Part model, mm, in its own coordinate system. Face numbers are marked on the shaded views. A direction names the side the tool comes from. Coordinates: 2 decimals unless noted, no trailing zeros. Loops run counter-clockwise (first coordinate to the right, second up) from the corner with the lowest first, then second, coordinate; pieces in that order, holes last. Notation, with made-up numbers: M 76.5,50.25 L 94.5,50.25 A10 ccw 94.5,68.25 Z; hole C 67.25,-1 d4. An arc over 180 degrees is marked long. Answer as CSV lines item,"result". Start each with the question number.
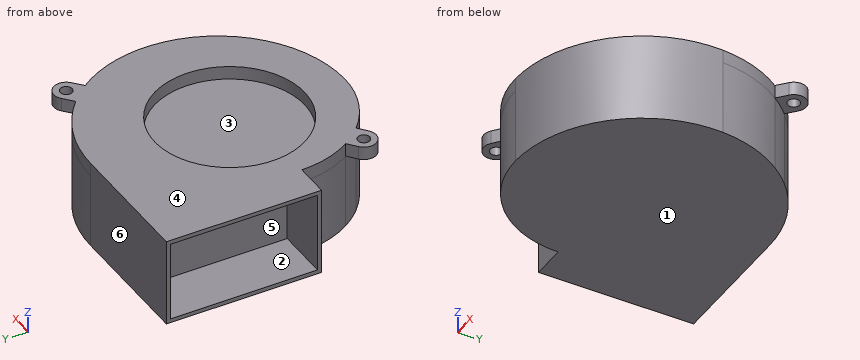
from build123d import *
from build123d.topology import SkipClean

# Parameters (mm, degrees)
SKETCH2_R           = 2.25
SKETCH2_R_2         = 28
BOSS_EXTRUDE1_DEPTH = 5
SKETCH5_R           = 28
BOSS_EXTRUDE3_DEPTH = 28
SKETCH6_W           = 30
SKETCH6_H           = 55
CUT_EXTRUDE1_DEPTH  = 20


with BuildPart() as part:
    # Sketch2 → Boss-Extrude1 (new body)
    # profile 1 of 3: a face of its own
    with BuildSketch(Plane.XY):
        with BuildLine():
            Line((35.933927487, 42.495954711), (32.250401879, 39.26537607))
            ThreePointArc((32.250401879, 39.26537607), (35.489083713, 35.92080567), (38.382546905, 32.273466648))
            Line((38.382546905, 32.273466648), (42.066072513, 35.504045289))
            ThreePointArc((42.066072513, 35.504045289), (42.495954711, 42.066072513), (35.933927487, 42.495954711))
        make_face()
        with Locations((39, 39)):
            Circle(SKETCH2_R, mode=Mode.SUBTRACT)
    # profile 2 of 3: a face of its own
    with BuildSketch(Plane.XY):
        with BuildLine():
            ThreePointArc((-25.556282339, -32.755867263), (-28.716218004, -29.331927128), (-31.420793753, -25.538007062))
            Line((-31.420793753, -25.538007062), (-34.932255707, -28.391069899))
            ThreePointArc((-34.932255707, -28.391069899), (-35.608930101, -34.932255707), (-29.067744293, -35.608930101))
            Line((-29.067744293, -35.608930101), (-25.556282339, -32.755867263))
        make_face()
        with Locations((-32, -32)):
            Circle(SKETCH2_R, mode=Mode.SUBTRACT)
    # profile 3 of 3: a face of its own
    with BuildSketch(Plane.XY):
        with BuildLine():
            ThreePointArc((0, -43), (-26.162950904, -32.162950904), (-37, -6))
            Line((-37, -6), (-50, -6))
            Line((-50, -6), (-50, 52))
            Line((-50, 52), (0, 52))
            ThreePointArc((0, 52), (32.250401879, 39.26537607), (47.1, 7.932509882))
            ThreePointArc((47.1, 7.932509882), (34.50998509, -27.669026021), (0, -43))
        make_face()
        Circle(SKETCH2_R_2, mode=Mode.SUBTRACT)
    extrude(amount=-BOSS_EXTRUDE1_DEPTH)

    # Sketch5 → Boss-Extrude3 (add)
    # profile 1 of 2: a face of its own
    with SkipClean():  # the faces are left unmerged after this step: merging them gives an invalid solid
        with BuildSketch(Plane.XY.offset(-5)):
            with BuildLine():
                ThreePointArc((32.250401879, 39.26537607), (17.336803829, 48.701069191), (0, 52))
                Line((0, 52), (-50, 52))
                Line((-50, 52), (-50, -6))
                Line((-50, -6), (-37, -6))
                ThreePointArc((-37, -6), (-35.577867902, -16.159493864), (-31.420793753, -25.538007062))
                ThreePointArc((-31.420793753, -25.538007062), (-28.716218004, -29.331927128), (-25.556282339, -32.755867263))
                ThreePointArc((-25.556282339, -32.755867263), (-13.766497581, -40.34360995), (0, -43))
                ThreePointArc((0, -43), (34.50998509, -27.669026021), (47.1, 7.932509882))
                ThreePointArc((47.1, 7.932509882), (44.44026328, 20.711463284), (38.382546905, 32.273466648))
                ThreePointArc((38.382546905, 32.273466648), (35.489083713, 35.92080567), (32.250401879, 39.26537607))
            make_face()
            Circle(SKETCH5_R, mode=Mode.SUBTRACT)
        # profile 2 of 2: a face of its own
        with BuildSketch(Plane.XY.offset(-5)):
            Circle(SKETCH5_R)
        extrude(amount=-BOSS_EXTRUDE3_DEPTH)

    # Sketch6 → Cut-Extrude1 (cut)
    with SkipClean():  # the faces are left unmerged after this step: merging them gives an invalid solid
        with BuildSketch(Plane.ZY.offset(50)):
            with Locations((-16.5, 23)):
                Rectangle(SKETCH6_W, SKETCH6_H)
        extrude(amount=-CUT_EXTRUDE1_DEPTH, mode=Mode.SUBTRACT)


solid = part.part
Q1. Flat gauge pins, fed straight in: P1, Ø9, axis at x = 37, y = 36, coming from the -Z side; P2, Ø5.5, axis at x = -30.5, y = -33.5, coming from the -Z side; P3, Ø4, axis at y = -2.5, z = -18.5, coming from the +X side; P4, Ø6, axis at x = 11.5, z = -15, coming from the +Y side. Where does each tip first touch, or does it go through?
Q2. Slice it at B-B, the plane y = 22.5. Write the cut outline in (x, z), and give its area (3 significant figures).
Q3. Slice it at A-A, the plane z = -7. Write the cut outline in (x, y), and give its area (3 significant figures).
Q4. Slice it at D-D, the plane y = -10. Write the cut outline in (x, z), and give its area (3 significant figures).
Q5. Tool access for the marked faces 1, 2 and 3: list every direction of +Z, -Z, +X, -X, +Y, -Y with a clear straight run to the whole face (end or side of a thin tool).
Q6. Wall check: L1, parallel to Y at x = 0, z = -2.9; L2, parallel to Z at x = -33.5, y = 45.5; L3, parallel to Y at x = -32, z = -1. Give the ranges that are in metal, low to high.
Q7. Slice it at C-C, the plane x = -20.5. Write the cut outline in (y, z).
Q8. Two-plate mould, pull along Y, no slides. Class the marked faces 4, 5 and 6: +Y half, -Y half, draft (parallel to the pull), parting line (faces both ways), or undercut.
Solved:
1,P1,"stops at z = -33"
1,P2,"stops at z = -5"
1,P3,"stops at x = 46.92"
1,P4,"stops at y = 51.23"
2,outline,"M -50,-33 L 43.76,-33 L 43.76,0 L 16.67,0 L 16.67,-5 L -16.67,-5 L -16.67,0 L -50,0 L -50,-1.5 L -30,-1.5 L -30,-31.5 L -50,-31.5 Z"
2,area,"2,330 mm2"
3,outline,"M -50,-6 L -37,-6 A37 ccw 0,-43 A47.76 ccw 47.1,7.93 A47.2 ccw 0,52 L -50,52 L -50,50.5 L -30,50.5 L -30,-4.5 L -50,-4.5 Z"
3,area,"6,390 mm2"
4,outline,"M -36.78,-33 L 44.87,-33 L 44.87,0 L 26.15,0 L 26.15,-5 L -26.15,-5 L -26.15,0 L -36.78,0 Z"
4,area,"2,430 mm2"
5,face 1,"-Z, +X, -X, +Y, -Y"
5,face 2,"-X"
5,face 3,"+Z"
6,L1,"y = -43 to -28, 28 to 52"
6,L2,"z = -33 to -31.5, -1.5 to 0"
6,L3,"y = -36.65 to -34.25, -29.75 to -26.01, -24.57 to 52"
7,outline,"M -36.8,-33 L 52,-33 L 52,0 L 19.07,0 L 19.07,-5 L -19.07,-5 L -19.07,0 L -36.8,0 Z"
8,face 4,"draft"
8,face 5,"undercut"
8,face 6,"+Y half"
